```python
from build123d import *

# Parameters (mm, degrees)
BOSS_EXTRUDE5_DEPTH = 19.8
SKETCH6_R           = 5.075
CUT_EXTRUDE1_DEPTH  = 10
FILLET2_R           = 0.5


with BuildPart() as part:
    # Sketch5 → Boss-Extrude5 (new body)
    with BuildSketch(Plane.XY):
        Polygon((4.330127019, 2.5), (1.443375673, 2.5), (-1.443375673, 2.5), (-2.886751346, 0), (-1.443375673, -2.5), (-2.886751346, -5), (-1.443375673, -7.5), (1.443375673, -7.5), (4.330127019, -7.5), (7.216878365, -7.5), (10.103629711, -7.5), (12.990381057, -7.5), (15.877132403, -7.5), (18.763883749, -7.5), (21.650635095, -7.5), (23.094010768, -5), (21.650635095, -2.5), (23.094010768, 0), (21.650635095, 2.5), (18.763883749, 2.5), (15.877132403, 2.5), (12.990381057, 2.5), (10.103629711, 2.5), (7.216878365, 2.5), align=None)
        Polygon((-0.866025404, -3.5), (0.866025404, -3.5), (2.020725942, -3.5), (19.341234018, -3.5), (21.073284825, -3.5), (21.939310229, -5), (21.073284825, -6.5), (19.341234018, -6.5), (0.866025404, -6.5), (-0.866025404, -6.5), (-1.732050808, -5), align=None, mode=Mode.SUBTRACT)
        Polygon((-0.866025404, 1.5), (0.866025404, 1.5), (18.186533479, 1.5), (19.341234018, 1.5), (21.073284825, 1.5), (21.939310229, 0), (21.073284825, -1.5), (19.341234018, -1.5), (0.866025404, -1.5), (-0.866025404, -1.5), (-1.732050808, 0), align=None, mode=Mode.SUBTRACT)
    extrude(amount=BOSS_EXTRUDE5_DEPTH)

    # Sketch6 → Cut-Extrude1 (cut)
    with BuildSketch(Plane.XZ.offset(7.5)):
        with Locations((10.103629827, 9.9)):
            Circle(SKETCH6_R)
    extrude(amount=-CUT_EXTRUDE1_DEPTH, mode=Mode.SUBTRACT)

    # Fillet2
    fillet2_edges = [part.edges().sort_by_distance(p)[0] for p in [
        (21.073284825, -3.5, 9.9),
        (-0.866025404, -3.5, 9.9),
        (-1.732050808, -5, 9.9),
        (-0.866025404, -6.5, 9.9),
        (21.073284825, -6.5, 9.9),
        (21.939310229, -5, 9.9),
        (21.650635095, 2.5, 9.9),
        (23.094010768, 0, 9.9),
        (21.650635095, -2.5, 9.9),
        (23.094010768, -5, 9.9),
        (21.650635095, -7.5, 9.9),
        (-1.443375673, -7.5, 9.9),
        (-2.886751346, -5, 9.9),
        (-1.443375673, -2.5, 9.9),
        (-2.886751346, 0, 9.9),
        (-1.443375673, 2.5, 9.9),
        (21.073284825, 1.5, 9.9),
        (-0.866025404, 1.5, 9.9),
        (-1.732050808, 0, 9.9),
        (-0.866025404, -1.5, 9.9),
        (21.073284825, -1.5, 9.9),
        (21.939310229, 0, 9.9),
    ]]
    fillet(fillet2_edges, radius=FILLET2_R)


solid = part.part
```
Design review of the part built by this model. Coordinates are the model's own, in mm. A direction names the side the tool comes from. Coordinates: 2 decimals unless noted, no trailing zeros. Loops run counter-clockwise (first coordinate to the right, second up) from the corner with the lowest first, then second, coordinate; pieces in that order, holes last. Notation, with made-up numbers: (61, 21) - (74, 21) arc R12 ccw to (74, 27) - close; hole circle Ø2 at (55, -17). An arc over 180 degrees is marked (long way). Use CSV: the item, a comma, the result in double quotes. Start each with the question number.
1) Consider section D-D on x = 6.75. Write out the cut boundary in (y, z), then the cut area to 3 significant figures.
2) Consider section A-A on x = 20. Write out the cut boundary in (y, z).
3) Wall thickness on L1, parallel to Y at x = 10.5, z = 15.75; L2, parallel to X at y = -6, z = 15.5; L3, parallel to X at y = -5.5, z = 2.25: over which ranges is each line inside the solid? List them lowest first. Write a range as from..to.
4) Consider section C-C on z = 16. Give the number of separate pieces and of enclosed holes in the cut face, then the cut area to 3 significant figures.
5) Tool access review of faces 4 (the flat face through (-2.17, -1.24, 9.76)), 5 (the flat face through (22.4, -3.8, 9.8)), 6 (the flat face through (21.5, 0.76, 9.76)), 7 (the flat face through (10, -2, 19.8)): name each direction out of +Z, -Z, +X, -X, +Y, -Y from which nothing blocks a thin tool from reaching the whole face with its end or side.
6) For pin 1 Ø6 at (x, z) = (10.5, 11.5) entering from -Y (1 decimal); pin 2 Ø5 at (x, y) = (11.5, -4.5) entering from +Z; pin 3 Ø2 at (y, z) = (-6.5, 12.5) entering from +X, all flat-tipped, find the tip position at first contact; note any pin that passes through.
7) Consider section B-B on x = 12.75. Write out the cut boundary in (y, z).
8) The part is to be moulded in two halves that separate along Y. For faces 1 (the flat face through (8, -3.5, 5)), 2 (the flat face through (-2.16, 1.26, 9.76)), 3 (the cylindrical face through (12.8, -7, 14.2)), say which applies: +Y half, -Y half, draft (parallel to the pull), parting line (faces both ways), or undercut.
Geometry says:
1,outline,"(-7.5, 0) - (-6.5, 0) - (-6.5, 6.09) - (-7.5, 6.09) - close; (-7.5, 13.71) - (-6.5, 13.71) - (-6.5, 19.8) - (-7.5, 19.8) - close; (-3.5, 0) - (-1.5, 0) - (-1.5, 6.09) - (-3.5, 6.09) - close; (-3.5, 13.71) - (-1.5, 13.71) - (-1.5, 19.8) - (-3.5, 19.8) - close; (1.5, 0) - (2.5, 0) - (2.5, 6.09) - (1.5, 6.09) - close; (1.5, 13.71) - (2.5, 13.71) - (2.5, 19.8) - (1.5, 19.8) - close"
1,area,"48.7 mm^2"
2,outline,"(-7.5, 0) - (-6.5, 0) - (-6.5, 19.8) - (-7.5, 19.8) - close; (-3.5, 0) - (-1.5, 0) - (-1.5, 19.8) - (-3.5, 19.8) - close; (1.5, 0) - (2.5, 0) - (2.5, 19.8) - (1.5, 19.8) - close"
3,L1,"-7.5..-6.5, -3.5..-1.5, 1.5..2.5"
3,L2,"-2.31..-1.15, 21.36..22.52"
3,L3,"-2.6..-1.44, 21.65..22.81"
4,separate pieces,"1"
4,enclosed holes,"2"
4,area,"109 mm^2"
5,face 4,"+Z, -Z, -X"
5,face 5,"+Z, -Z, +X"
5,face 6,"+Z, -Z"
5,face 7,"+Z, +X, -X, +Y, -Y"
6,pin 1,"through"
6,pin 2,"z = 19.8"
6,pin 3,"x = 22.81"
7,outline,"(-7.5, 0) - (-6.5, 0) - (-6.5, 5.57) - (-7.5, 5.57) - close; (-7.5, 14.23) - (-6.5, 14.23) - (-6.5, 19.8) - (-7.5, 19.8) - close; (-3.5, 0) - (-1.5, 0) - (-1.5, 5.57) - (-3.5, 5.57) - close; (-3.5, 14.23) - (-1.5, 14.23) - (-1.5, 19.8) - (-3.5, 19.8) - close; (1.5, 0) - (2.5, 0) - (2.5, 5.57) - (1.5, 5.57) - close; (1.5, 14.23) - (2.5, 14.23) - (2.5, 19.8) - (1.5, 19.8) - close"
8,face 1,"undercut"
8,face 2,"+Y half"
8,face 3,"draft"
